Can you work these out from the model? Positions are in its coordinate system, mm. A direction names the side the tool comes from. Coordinates: 2 decimals unless noted, no trailing zeros. Loops run counter-clockwise (first coordinate to the right, second up) from the corner with the lowest first, then second, coordinate; pieces in that order, holes last.
```python
from build123d import *

# Parameters (mm, degrees)
F0_R           = 3.3
F1_DEPTH       = 5
F2_D           = 6.6
F2_DEPTH       = 20
F2_CBORE_D     = 11.25
F2_CBORE_DEPTH = 2


with BuildPart() as f1:
    # F0 (on Front) → F1 (new body)
    with BuildSketch(Plane.XZ):
        Polygon((0, 65), (0, 0), (28, 0), (28, 10), (55, 37), (65, 37), (65, 65), align=None)
        with Locations((14, 10)):
            Circle(F0_R, mode=Mode.SUBTRACT)
        with Locations((14, 51)):
            Circle(F0_R, mode=Mode.SUBTRACT)
        with Locations((55, 51)):
            Circle(F0_R, mode=Mode.SUBTRACT)
    extrude(amount=-F1_DEPTH)

    # F2
    with Locations(Plane.XZ):
        with Locations((14, 51), (55, 51), (14, 10)):
            CounterBoreHole(F2_D / 2, F2_CBORE_D / 2, F2_CBORE_DEPTH, depth=F2_DEPTH)


solid = f1.part
```
(1) I'm going to push flat-ended pins straight in: pin 1 (1.5 mm diameter, centred on y = 1.5, z = 6.5, fed in from +X); pin 2 (10 mm diameter, centred on x = 14, z = 10, fed in from -Y); pin 3 (1.5 mm diameter, centred on x = 61, y = 3.5, fed in from -Z). Where does each tip first touch, or does it pass through?
Check values:
pin 1: stops at x = 28
pin 2: stops at y = 2
pin 3: stops at z = 37
(2) I want a section at A-A on y = 2.75. Write out the boundary of the cut face in (x, z), then the cut area to 3 significant figures.
Check values:
outline: (0, 0) - (28, 0) - (28, 10) - (55, 37) - (65, 37) - (65, 65) - (0, 65) - close; hole circle Ø6.6 at (14, 10); hole circle Ø6.6 at (14, 51); hole circle Ø6.6 at (55, 51)
area: 3,120 mm2
(3) Which directions (+Z, -Z, +X, -X, +Y, -Y) give clear straight access to the entire face, cutting with the end or side of a thin tool? Please do faces 1 (the flat face through (25, 5, 40)), 2 (the flat face through (14, 2, 47)), 3 (the flat face through (28, 2, 5)).
Check values:
face 1: +Z, -Z, +X, -X, +Y
face 2: -Y
face 3: -Z, +X, +Y, -Y
(4) I want a section at C-C on x = 14. Write out the boundary of the cut face in (y, z) (3 decimals).
Check values:
outline: (0, 0) - (5, 0) - (5, 6.7) - (2, 6.7) - (2, 4.375) - (0, 4.375) - close; (0, 15.625) - (2, 15.625) - (2, 13.3) - (5, 13.3) - (5, 47.7) - (2, 47.7) - (2, 45.375) - (0, 45.375) - close; (0, 56.625) - (2, 56.625) - (2, 54.3) - (5, 54.3) - (5, 65) - (0, 65) - close
(5) I want a section at D-D on x = 53.5. Write out the boundary of the cut face in (y, z), then the cut area to 3 significant figures.
Check values:
outline: (0, 35.5) - (5, 35.5) - (5, 48.06) - (2, 48.06) - (2, 45.58) - (0, 45.58) - close; (0, 56.42) - (2, 56.42) - (2, 53.94) - (5, 53.94) - (5, 65) - (0, 65) - close
area: 108 mm2
(6) I want a section at B-B on z = 51. Write out the boundary of the cut face in (x, y) (3 decimals), then the cut area to 3 significant figures.
Check values:
outline: (0, 0) - (8.375, 0) - (8.375, 2) - (10.7, 2) - (10.7, 5) - (0, 5) - close; (17.3, 2) - (19.625, 2) - (19.625, 0) - (49.375, 0) - (49.375, 2) - (51.7, 2) - (51.7, 5) - (17.3, 5) - close; (58.3, 2) - (60.625, 2) - (60.625, 0) - (65, 0) - (65, 5) - (58.3, 5) - close
area: 240 mm2
(7) If we mould it in two halves opening along X, with no side actions, what happens to faces 4 (the flat face through (55, 2, 47)), 5 (the flat face through (65, 2, 51)), 6 (the flat face through (60, 2, 37))? For each: released by +X, released by -X, zero draft, split by the parting line, or undercut.
Check values:
face 4: undercut
face 5: released by +X
face 6: zero draft
(8) If I drill on probe 1 along Z at (x, y) = (55, 3.1); probe 2 along X at (y, z) = (0.85, 55.5) (3 decimals); probe 3 along X at (y, z) = (1.8, 47), over which ranges is the centre line in solid material (lowest first)?
Check values:
probe 1: z = 37 to 47.7, 54.3 to 65
probe 2: x = 0 to 10.625, 17.375 to 51.625, 58.375 to 65
probe 3: x = 0 to 10.05, 17.95 to 51.05, 58.95 to 65
